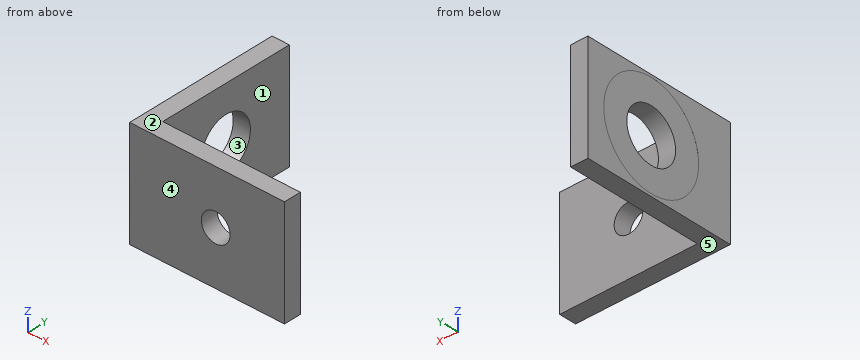
```python
from build123d import *

# Parameters (mm, degrees)
BOSS_EXTRUDE1_DEPTH     = 20
F_3_8_CLEARANCE_HOLE1_D = 9.8044
M5_CLEARANCE_HOLE1_D    = 5.3
SKETCH2_R               = 9.525
CUT_EXTRUDE1_DEPTH      = 0.001


with BuildPart() as part:
    # Sketch1 → Boss-Extrude1 (new body)
    with BuildSketch(Plane.XY):
        Polygon((0, 2.54), (0, 25.4), (-3.175, 25.4), (-3.175, -3.175), (25.4, -3.175), (25.4, 0), (2.54, 0), (0, 0), align=None)
    extrude(amount=BOSS_EXTRUDE1_DEPTH)

    # 3/8 Clearance Hole1 (through all)
    with Locations(Plane.ZY.offset(3.175)):
        with Locations((10, 12.7)):
            Hole(F_3_8_CLEARANCE_HOLE1_D / 2)

    # M5 Clearance Hole1 (through all)
    with Locations(Plane(origin=(0, 0, 0), x_dir=(1, 0, 0), z_dir=(0, 1, 0))):
        with Locations((12.7, -10)):
            Hole(M5_CLEARANCE_HOLE1_D / 2)

    # Sketch2 → Cut-Extrude1 (cut)
    with BuildSketch(Plane.ZY.offset(3.175)):
        with Locations((10, 12.7)):
            Circle(SKETCH2_R)
    extrude(amount=-CUT_EXTRUDE1_DEPTH, mode=Mode.SUBTRACT)


solid = part.part
```
Verification items for the finished model (mm, model axes). Face numbers are marked on the shaded views. A direction names the side the tool comes from. Round coordinates to 2 decimals unless told otherwise and drop trailing zeros. Order: outer loops, then holes, each group sorted by start corner. A loop starts at its lowest first (then second) coordinate and runs counter-clockwise, first axis right, second up. Notation, with made-up numbers: (-24.5, -14.5) -> (20.5, -14.5) arc R20 cw to (20.5, 6.5) -> close; hole circle Ø9 at (-17.75, 68). An arc over 180 degrees is marked (long way). Put each result on its own line as item: value. Start each with the question number.
(1) Draft check along Z on the marked faces 3, 4 and 5. Enter one of: +Z half, -Z half, draft (parallel to the pull), parting line (faces both ways), or undercut.
(2) Material ranges on line 1 along Y through (x, z) = (-1.35, 10) (3 decimals); line 2 along X through (y, z) = (-2.4, 10) (3 decimals); line 3 along Y through (x, z) = (22.75, 10.75) (3 decimals), recorded low to high.
(3) Section check D-D (y = -0.5). Enter the section's corners in (x, z) (3 decimals).
(4) Section check C-C (z = 9). State how many separate pieces and enclosed holes the cut face has, then the cut area to 3 significant figures.
(5) Depth check by flat-ended pin: pin 1 Ø10 at (x, z) = (10.5, 10) entering from +Y. Enter the tip coordinate at first touch or a pass-through.
(6) Section check B-B (x = 12.7). Enter the section's corners in (y, z) (3 decimals).
(7) Tool access check on the marked faces 1 and 2. Record the directions out of +Z, -Z, +X, -X, +Y, -Y that give a thin tool (end or side, any length) a straight path to the whole face; none if there is none.
Completed:
1. face 3: undercut
1. face 4: draft
1. face 5: -Z half
2. line 1: y = -3.175 to 7.798, 17.602 to 25.4
2. line 2: x = -3.175 to 10.05, 15.35 to 25.4
2. line 3: y = -3.175 to 0
3. outline: (-3.175, 0) -> (25.4, 0) -> (25.4, 20) -> (-3.175, 20) -> close; hole circle Ø5.3 at (12.7, 10)
4. separate pieces: 3
4. enclosed holes: 0
4. area: 125 mm2
5. pin 1: stops at y = 0
6. outline: (-3.175, 0) -> (0, 0) -> (0, 7.35) -> (-3.175, 7.35) -> close; (-3.175, 12.65) -> (0, 12.65) -> (0, 20) -> (-3.175, 20) -> close
7. face 1: +Z, -Z, +X, +Y
7. face 2: +Z, +X, -X, +Y, -Y
